```python
from build123d import *

# Parameters (mm, degrees)
SKETCH1_W                      = 65
SKETCH1_H                      = 50
BASE_FLANGE1_DEPTH             = 3
EDGE_FLANGE1_STRIP_W           = 21
EDGE_FLANGE1_STRIP_H           = 3
EDGE_FLANGE1_STRIP_CUT_DEPTH   = 50
EDGE_FLANGE1_STRIP_2_W         = 21
EDGE_FLANGE1_STRIP_2_H         = 3
EDGE_FLANGE1_STRIP_CUT_2_DEPTH = 50
EDGE_FLANGE1_DEPTH             = 50
EDGE_FLANGE1_BEND_DEPTH        = 50
SKETCH13_R                     = 2.5
CUT_EXTRUDE1_DEPTH             = 10
SKETCH14_W                     = 20
SKETCH14_H                     = 3
BOSS_EXTRUDE1_DEPTH            = 18
FILLET1_R                      = 9.5
SKETCH15_R                     = 3
CUT_EXTRUDE2_DEPTH             = 31


# Sheet-metal steps are written as plain solids
with BuildPart() as part:
    # Sketch1 → Base-Flange1 (new body)
    with BuildSketch(Plane.YZ):
        Rectangle(SKETCH1_W, SKETCH1_H)
    extrude(amount=BASE_FLANGE1_DEPTH)

    # Edge-Flange1 strip (across the edge) → Edge-Flange1 strip cut (cut)
    with BuildSketch(Plane(origin=(0, 32.5, 25), x_dir=(0, -1, 0), z_dir=(0, 0, -1))):
        with Locations((-6, -1.5)):
            Rectangle(EDGE_FLANGE1_STRIP_W, EDGE_FLANGE1_STRIP_H)
    extrude(amount=EDGE_FLANGE1_STRIP_CUT_DEPTH, mode=Mode.SUBTRACT)

    # Edge-Flange1 strip 2 (across the edge) → Edge-Flange1 strip cut 2 (cut)
    with BuildSketch(Plane(origin=(0, -32.5, -25), x_dir=(0, 1, 0), z_dir=(0, 0, 1))):
        with Locations((-6, -1.5)):
            Rectangle(EDGE_FLANGE1_STRIP_2_W, EDGE_FLANGE1_STRIP_2_H)
    extrude(amount=EDGE_FLANGE1_STRIP_CUT_2_DEPTH, mode=Mode.SUBTRACT)

    # Edge-Flange1 section (across the edge) → Edge-Flange1 (add)
    with BuildSketch(Plane(origin=(0, 32.5, 25), x_dir=(0, -1, 0), z_dir=(0, 0, -1))):
        with BuildLine():
            Line((-3, 4.5), (-3, 17))
            Line((-3, 17), (0, 17))
            Line((0, 17), (0, 4.5))
            ThreePointArc((0, 4.5), (1.318019485, 1.318019485), (4.5, 0))
            Line((4.5, 0), (4.5, -3))
            ThreePointArc((4.5, -3), (-0.803300859, -0.803300859), (-3, 4.5))
        make_face()
    extrude(amount=EDGE_FLANGE1_DEPTH)

    # Edge-Flange1 section 2 (across the edge) → Edge-Flange1 bend (add)
    with BuildSketch(Plane(origin=(0, -32.5, -25), x_dir=(0, 1, 0), z_dir=(0, 0, 1))):
        with BuildLine():
            Line((-3, 4.5), (-3, 17))
            Line((-3, 17), (0, 17))
            Line((0, 17), (0, 4.5))
            ThreePointArc((0, 4.5), (1.318019485, 1.318019485), (4.5, 0))
            Line((4.5, 0), (4.5, -3))
            ThreePointArc((4.5, -3), (-0.803300859, -0.803300859), (-3, 4.5))
        make_face()
    extrude(amount=EDGE_FLANGE1_BEND_DEPTH)

    # Sketch13 → Cut-Extrude1 (cut)
    with BuildSketch(Plane.YZ.offset(3)):
        with Locations(Location((-17, 15, 0), (0, 0, 270))):
            Circle(SKETCH13_R)
        with Locations(Location((17, 15, 0), (0, 0, 270))):
            Circle(SKETCH13_R)
    extrude(amount=-CUT_EXTRUDE1_DEPTH, mode=Mode.SUBTRACT)

    # Sketch14 → Boss-Extrude1 (add)
    with BuildSketch(Plane.YZ.offset(3)):
        with Locations((0, 11.5)):
            Rectangle(SKETCH14_W, SKETCH14_H)
        with Locations((0, -11.5)):
            Rectangle(SKETCH14_W, SKETCH14_H)
    extrude(amount=BOSS_EXTRUDE1_DEPTH)

    # Fillet1
    fillet1_edges = [part.edges().sort_by_distance(p)[0] for p in [
        (21, -10, 11.5),
        (21, 10, 11.5),
        (21, -10, -11.5),
        (21, 10, -11.5),
    ]]
    fillet(fillet1_edges, radius=FILLET1_R)

    # Sketch15 → Cut-Extrude2 (cut)
    with BuildSketch(Plane.XY.offset(13)):
        with Locations((11, 0)):
            Circle(SKETCH15_R)
    extrude(amount=-CUT_EXTRUDE2_DEPTH, mode=Mode.SUBTRACT)


solid = part.part
```
Part model, mm, in its own coordinate system. A direction names the side the tool comes from. Round coordinates to 2 decimals unless told otherwise and drop trailing zeros. Write each loop counter-clockwise with the first axis right and the second up, starting at its lowest first coordinate (ties: lowest second). Pieces come first, ordered by that corner, then holes. Notation, with made-up numbers: M 79.25,30.5 L 130.25,30.5 A20 ccw 130.25,67.5 Z; hole C -37.75,-31 d2. An arc over 180 degrees is marked long. One line per question, with ' | ' between items.
(1) Saw through at C-C on x = -8. Write the cut outline in (y, z).
Answer key:
outline: M -35.5,-25 L -32.5,-25 L -32.5,25 L -35.5,25 Z; M 32.5,-25 L 35.5,-25 L 35.5,25 L 32.5,25 Z
(2) Saw through at A-A on y = 18.5. Write the cut outline in (x, z), then the cut area to 3 significant figures.
Answer key:
outline: M 0,-25 L 3,-25 L 3,13 L 0,13 Z; M 0,17 L 3,17 L 3,25 L 0,25 Z | area: 138 mm^2
(3) Pin check, flat tips, straight feed: pin 1 (3.5 mm diameter, centred on x = 7.5, z = 11.5, fed in from +Y); pin 2 (5 mm diameter, centred on x = 11, y = 0, fed in from -Z); pin 3 (3 mm diameter, centred on y = 17.5, z = 19, fed in from +X); pin 4 (3.5 mm diameter, centred on x = 7.5, z = 12, fed in from -Y). Stop position of each tip, or through.
Answer key:
pin 1: stops at y = 10 | pin 2: passes through | pin 3: stops at x = 3 | pin 4: stops at y = -10
(4) Saw through at B-B on z = 15. Write the cut outline in (x, y).
Answer key:
outline: M -17,-35.5 L -4.5,-35.5 A7.5 ccw 3,-28 L 3,-19.5 L 0,-19.5 L 0,-28 A4.5 cw -4.5,-32.5 L -17,-32.5 Z; M -17,32.5 L -4.5,32.5 A4.5 cw 0,28 L 0,19.5 L 3,19.5 L 3,28 A7.5 ccw -4.5,35.5 L -17,35.5 Z; M 0,-14.5 L 3,-14.5 L 3,14.5 L 0,14.5 Z
(5) 3-axis set-ups, long thin cutter, end or side, ignore diameter. For faces 4 (the face through (7, -10, 11)), 5 (the face through (14, 2, 10)), 6 (the face through (-1.353, -31.217, -0.35)): which of +Z, -Z, +X, -X, +Y, -Y reach the whole face in a straight line?
Answer key:
face 4: +Z, -Z, +X, -Y | face 5: +X, +Y, -Y | face 6: +Z, -Z, -X
(6) Saw through at D-D on z = 7. Write the cut outline in (x, y), then the cut area to 3 significant figures.
Answer key:
outline: M -17,-35.5 L -4.5,-35.5 A7.5 ccw 3,-28 L 3,28 A7.5 ccw -4.5,35.5 L -17,35.5 L -17,32.5 L -4.5,32.5 A4.5 cw 0,28 L 0,-28 A4.5 cw -4.5,-32.5 L -17,-32.5 Z | area: 300 mm^2
(7) Two-plate mould, pull along Y, no slides. Class faces 1 (the face through (0.4, 0.2, -25)), 2 (the face through (18.143, 7.291, -11.479)), 3 (the face through (-1.353, 31.217, 0.35)): released by +Y, released by -Y, zero draft, split by the parting line, or undercut.
Answer key:
face 1: zero draft | face 2: released by +Y | face 3: undercut
(8) Probe line 1 along Y through (x, z) = (-8, -16.5); line 2 along Z through (x, y) = (5, 1.5); line 3 along Y through (x, z) = (1.75, 15). List the from-to ranges inside material, lowest first.
Answer key:
line 1: y = -35.5 to -32.5, 32.5 to 35.5 | line 2: z = -13 to -10, 10 to 13 | line 3: y = -32.15 to -19.5, -14.5 to 14.5, 19.5 to 32.15
